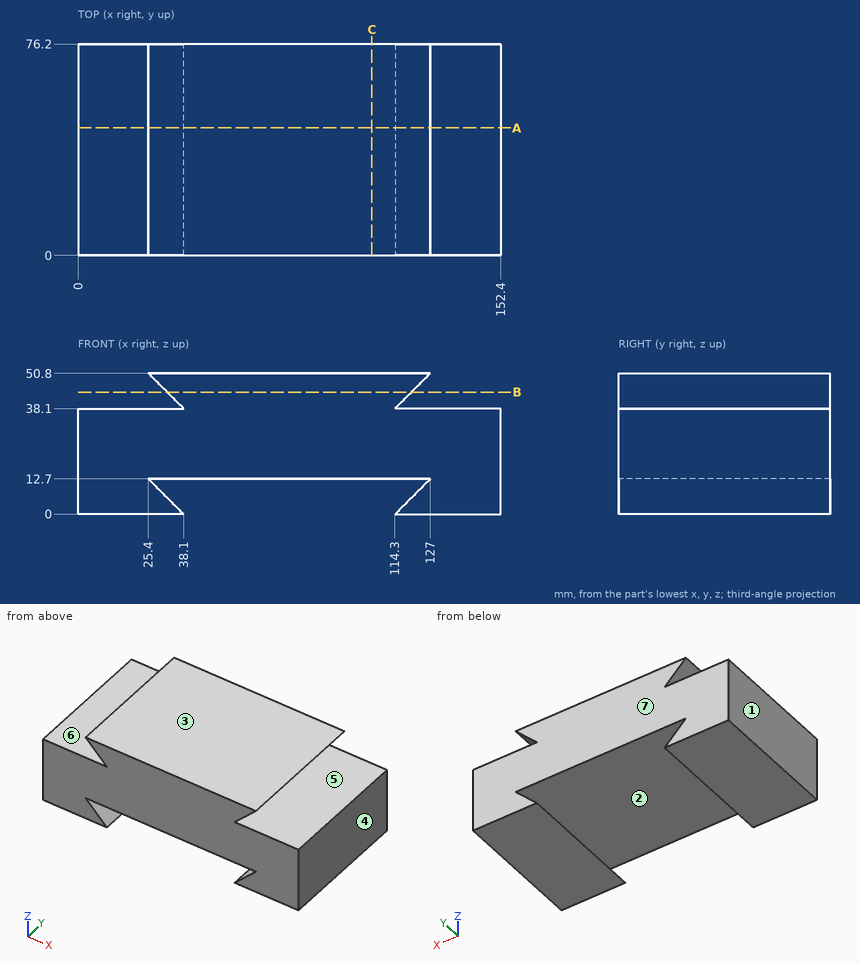
Source: three-view drawing plus pictorial views. Frame: mm from the lowest corner of the part. A direction names the side the tool comes from. Coordinates: 2 decimals unless noted, no trailing zeros. Order: outer loops, then holes, each group sorted by start corner. A loop starts at its lowest first (then second) coordinate and runs counter-clockwise, first axis right, second up. Notation, with made-up numbers: M -39,63 L 19,63 A21 cw 19,70 Z; hole C 48,-20.5 d2. An arc over 180 degrees is marked long. Answer in a Markdown table with one row per item.
(1) Access query for the marked faces 5, 6 and 7. Directions: +Z, -Z, +X, -X, +Y, -Y. A direction counts if a zero-diameter tool reaches every point of the face in a straight line with its end or side. Return the directions, or none.
Numbers:
| item | result |
|---|---|
| face 5 | +X, +Y, -Y |
| face 6 | -X, +Y, -Y |
| face 7 | +Z, -Z, +X, -X, +Y |
(2) Material intervals for line 1 (Z direction, x = 125, y = 42); line 2 (Z direction, x = 15.5, y = 72); line 3 (Z direction, x = 68, y = 55.5), sorted ascending. Write a range as [from, to].
Numbers:
| item | result |
|---|---|
| line 1 | z = [0, 10.7], [12.7, 38.1], [48.8, 50.8] |
| line 2 | z = [0, 38.1] |
| line 3 | z = [12.7, 50.8] |
(3) Draft query along X for the marked faces 1, 2, 3 and 4. Return one class per face: pulls with the +X half, pulls with the -X half, needs draft (parallel to the pull), parting line crosses it, or undercut.
Numbers:
| item | result |
|---|---|
| face 1 | pulls with the -X half |
| face 2 | undercut |
| face 3 | needs draft |
| face 4 | pulls with the +X half |
(4) Section query A-A, the plane y = 46. Output: boundary loops of the cut face in (x, z), plus the area to 3 significant figures.
Numbers:
| item | result |
|---|---|
| outline | M 0,0 L 38.1,0 L 25.4,12.7 L 127,12.7 L 114.3,0 L 152.4,0 L 152.4,38.1 L 114.3,38.1 L 127,50.8 L 25.4,50.8 L 38.1,38.1 L 0,38.1 Z |
| area | 5,810 mm^2 |
(5) Contact query for flat-ended pins moving along their axis: pin 1 Ø10 at (y, z) = (58.5, 45.5) entering from +X; pin 2 Ø11.5 at (x, y) = (139, 51.5) entering from +Z; pin 3 Ø6 at (x, z) = (81.5, 26) entering from -Y; pin 4 Ø1 at (y, z) = (39.5, 41.5) entering from +X. Output: stop coordinate, or through.
Numbers:
| item | result |
|---|---|
| pin 1 | stops at x = 126.7 |
| pin 2 | stops at z = 38.1 |
| pin 3 | stops at y = 0 |
| pin 4 | stops at x = 118.2 |
(6) Section query B-B, the plane z = 44. Output: boundary loops of the cut face in (x, y).
Numbers:
| item | result |
|---|---|
| outline | M 32.2,0 L 120.2,0 L 120.2,76.2 L 32.2,76.2 Z |
(7) Section query C-C, the plane x = 106. Output: boundary loops of the cut face in (y, z).
Numbers:
| item | result |
|---|---|
| outline | M 0,12.7 L 76.2,12.7 L 76.2,50.8 L 0,50.8 Z |
